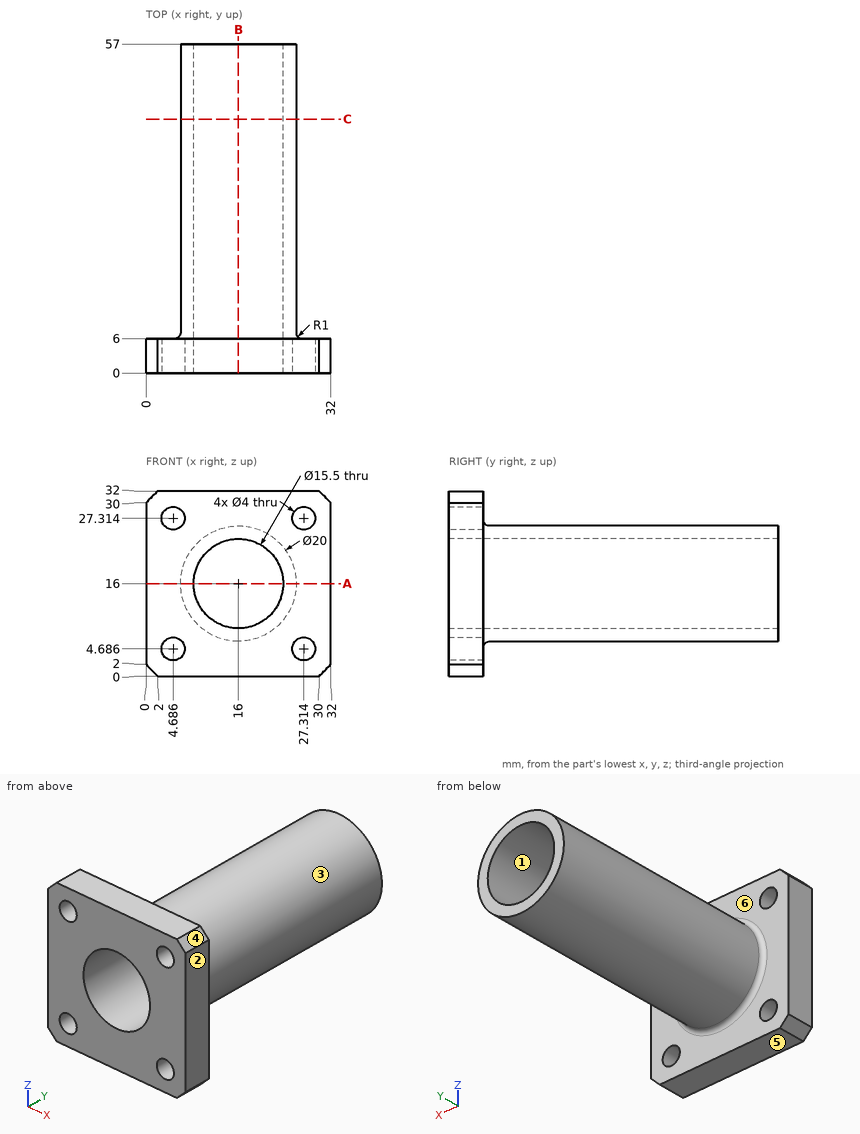
Study the drawing (mm; zero at the part's minimum x, y, z) and answer. A direction names the side the tool comes from. Round coordinates to 2 decimals unless told otherwise and drop trailing zeros. Write each loop counter-clockwise with the first axis right and the second up, starting at its lowest first coordinate (ties: lowest second). Pieces come first, ordered by that corner, then holes. Notation, with made-up numbers: (21, -27) - (36, -27) arc R29 ccw to (36, -4) - close; hole circle Ø8 at (36.5, 56). An arc over 180 degrees is marked (long way). Use a Markdown table: item, result. Add a question column.
1. A tool of negligible diameter and unlimited length cuts with its end or side. For the marked faces 5 and 6, from which of +Z, -Z, +X, -X, +Y, -Y can it reach the whole face along a straight path? Write none if from no direction.
2. The part is cut by section A-A (z = 16). Write down the section's boundary in (x, y), and give its area (3 significant figures).
3. Flat-ended cylindrical pins translate along their axes: P1, Ø3.5, axis at x = 27.31, z = 27.31, coming from the -Y side; P2, Ø5, axis at x = 12.5, y = 36, coming from the +Z side; P3, Ø8, axis at y = 16.5, z = 17.5, coming from the +X side; P4, Ø1.5, axis at x = 21.5, y = 47, coming from the -Z side. Find the tip coordinate at first contact, or state that the pin passes through.
4. The part is cut by section B-B (x = 16). Write down the section's boundary in (y, z).
5. For a pull along Z with two mould halves and no side action, classify the marked faces 1, 2, 3 and 4 as +Z half, -Z half, draft (parallel to the pull), parting line (faces both ways), or undercut.
6. The part is cut by section C-C (y = 44). Write down the section's boundary in (x, z).
7. Consider line 1 (X direction, y = 11.5, z = 16); line 2 (Y direction, x = 21, z = 26.5); line 3 (X direction, y = 29.5, z = 12.5) (1 decimal). Determine where each line is inside the solid, lowest interval first.
Reported:
| question | item | result |
|---|---|---|
| 1 | face 5 | -Z, +X, -X, +Y, -Y |
| 1 | face 6 | +Y |
| 2 | outline | (0, 0) - (8.25, 0) - (8.25, 57) - (6, 57) - (6, 7) arc R1 cw to (5, 6) - (0, 6) - close; (23.75, 0) - (32, 0) - (32, 6) - (27, 6) arc R1 cw to (26, 7) - (26, 57) - (23.75, 57) - close |
| 2 | area | 329 mm^2 |
| 3 | P1 | through |
| 3 | P2 | z = 25.95 |
| 3 | P3 | x = 26 |
| 3 | P4 | z = 7.2 |
| 4 | outline | (0, 0) - (6, 0) - (6, 5) arc R1 cw to (7, 6) - (57, 6) - (57, 8.25) - (0, 8.25) - close; (0, 23.75) - (57, 23.75) - (57, 26) - (7, 26) arc R1 cw to (6, 27) - (6, 32) - (0, 32) - close |
| 5 | face 1 | undercut |
| 5 | face 2 | draft |
| 5 | face 3 | parting line |
| 5 | face 4 | +Z half |
| 6 | outline | circle Ø20 at (16, 16); hole circle Ø15.5 at (16, 16) |
| 7 | line 1 | 6 to 8.25, 23.75 to 26 |
| 7 | line 2 | 0 to 6 |
| 7 | line 3 | 6.6 to 9.1, 22.9 to 25.4 |
